from build123d import *

# Parameters (mm, degrees)
SKETCH1_W           = 11.6
SKETCH1_H           = 10.6
BOSS_EXTRUDE1_DEPTH = 2
SKETCH2_R           = 0.85805849
SKETCH2_R_2         = 0.505403016
CUT_EXTRUDE1_DEPTH  = 9.107404023


with BuildPart() as part:
    # Sketch1 → Boss-Extrude1 (new body)
    with BuildSketch(Plane(origin=(0, 0, 0), x_dir=(1, 0, 0), z_dir=(0, 1, 0))):
        Rectangle(SKETCH1_W, SKETCH1_H)
    extrude(amount=BOSS_EXTRUDE1_DEPTH)

    # Sketch2 → Cut-Extrude1 (cut, through all)
    with BuildSketch(Plane(origin=(0, 2, 0), x_dir=(1, 0, 0), z_dir=(0, 1, 0))):
        with Locations(Location((-3.600453249, 0.480060433, 0), (0, 0, 270))):
            Circle(SKETCH2_R)
        with Locations(Location((0.029546751, 0.480060433, 0), (0, 0, 270))):
            Circle(SKETCH2_R)
        with Locations(Location((3.659546751, 0.480060433, 0), (0, 0, 270))):
            Circle(SKETCH2_R)
        with Locations(Location((-5.040634548, -4.35610393, 0), (0, 0, 270))):
            Circle(SKETCH2_R_2)
        with Locations(Location((-3.000634548, -4.35610393, 0), (0, 0, 270))):
            Circle(SKETCH2_R_2)
        with Locations(Location((-0.960634548, -4.35610393, 0), (0, 0, 270))):
            Circle(SKETCH2_R_2)
        with Locations(Location((1.079365452, -4.35610393, 0), (0, 0, 270))):
            Circle(SKETCH2_R_2)
        with Locations(Location((3.119365452, -4.35610393, 0), (0, 0, 270))):
            Circle(SKETCH2_R_2)
        with Locations(Location((5.159365452, -4.35610393, 0), (0, 0, 270))):
            Circle(SKETCH2_R_2)
        with BuildLine():
            Line((-5.8, 0.960120866), (-5.8, 5.3))
            Line((-5.8, 5.3), (-3.19151288, 5.3))
            ThreePointArc((-3.19151288, 5.3), (-5.039424989, 3.456832761), (-5.8, 0.960120866))
        make_face()
        with BuildLine():
            Line((3.120392815, 5.3), (5.8, 5.3))
            Line((5.8, 5.3), (5.8, 0.960120866))
            ThreePointArc((5.8, 0.960120866), (5.008377062, 3.468528113), (3.120392815, 5.3))
        make_face()
    extrude(amount=-CUT_EXTRUDE1_DEPTH, mode=Mode.SUBTRACT)


solid = part.part
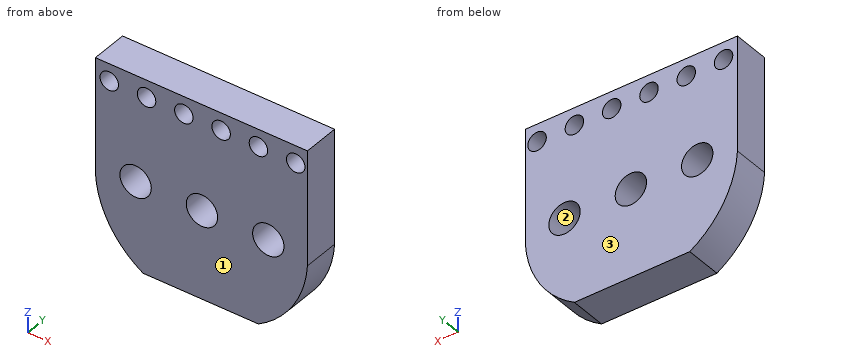
Geometry check sheet. Reference: the model listing, model coordinates, mm. Face numbers are marked on the shaded views. Give positions to 0.01 mm unless a question says otherwise; leave off trailing zeros. Order: outer loops, then holes, each group sorted by start corner. A loop starts at its lowest first (then second) coordinate and runs counter-clockwise, first axis right, second up. Notation, with made-up numbers: (89, 5) - (127, 5) arc R22 cw to (127, 19) - close; hole circle Ø7 at (69.5, 69.25). An arc over 180 degrees is marked (long way). Use one line per item in the form item = value.
1) Depth check by flat-ended pin: pin 1 Ø1.4 at (x, z) = (0.03, -0.48) entering from +Y; pin 2 Ø1 at (y, z) = (1.5, -2) entering from -X. Enter the tip coordinate at first touch or a pass-through.
Working result:
pin_1 = through
pin_2 = -5.75
2) Sectioned sample at D-D (z = -4). Record the boundary of the cut face in (x, y).
Working result:
outline = (-4.67, 0) - (4.63, 0) - (4.63, 2) - (-4.67, 2) - close
3) Draft check along Y on the marked faces 1, 2 and 3. Enter one of: released by +Y, released by -Y, zero draft, split by the parting line, or undercut.
Working result:
face_1 = released by -Y
face_2 = zero draft
face_3 = released by +Y
4) Sectioned sample at B-B (x = -4.75). Record the boundary of the cut face in (y, z), and give its area (3 significant figures).
Working result:
outline = (0, -3.89) - (2, -3.89) - (2, 3.94) - (0, 3.94) - close; (0, 4.77) - (2, 4.77) - (2, 5.3) - (0, 5.3) - close
area = 16.7 mm^2
5) Sectioned sample at C-C (y = 0.35). Count the separate pieces of the cut face and the enclosed holes in it, and give its area (3 significant figures).
Working result:
separate_pieces = 1
enclosed_holes = 9
area = 104 mm^2
6) Sectioned sample at A-A (z = 0.25). Record the boundary of the cut face in (x, y).
Working result:
outline = (-5.8, 0) - (-4.05, 0) - (-4.05, 2) - (-5.8, 2) - close; (-3.15, 0) - (-0.42, 0) - (-0.42, 2) - (-3.15, 2) - close; (0.48, 0) - (3.21, 0) - (3.21, 2) - (0.48, 2) - close; (4.11, 0) - (5.8, 0) - (5.8, 2) - (4.11, 2) - close
7) Material ranges on probe 1 along Z at (x, y) = (3.5, 1.2); probe 2 along Z at (x, y) = (-4.75, 0.95); probe 3 along Z at (x, y) = (-0.75, 0.7), recorded low to high. Write a range as from..to.
Working result:
probe_1 = -5.06..-1.32, 0.36..4.02, 4.69..5.3
probe_2 = -3.89..3.94, 4.77..5.3
probe_3 = -5.3..-0.84, -0.12..3.9, 4.82..5.3
